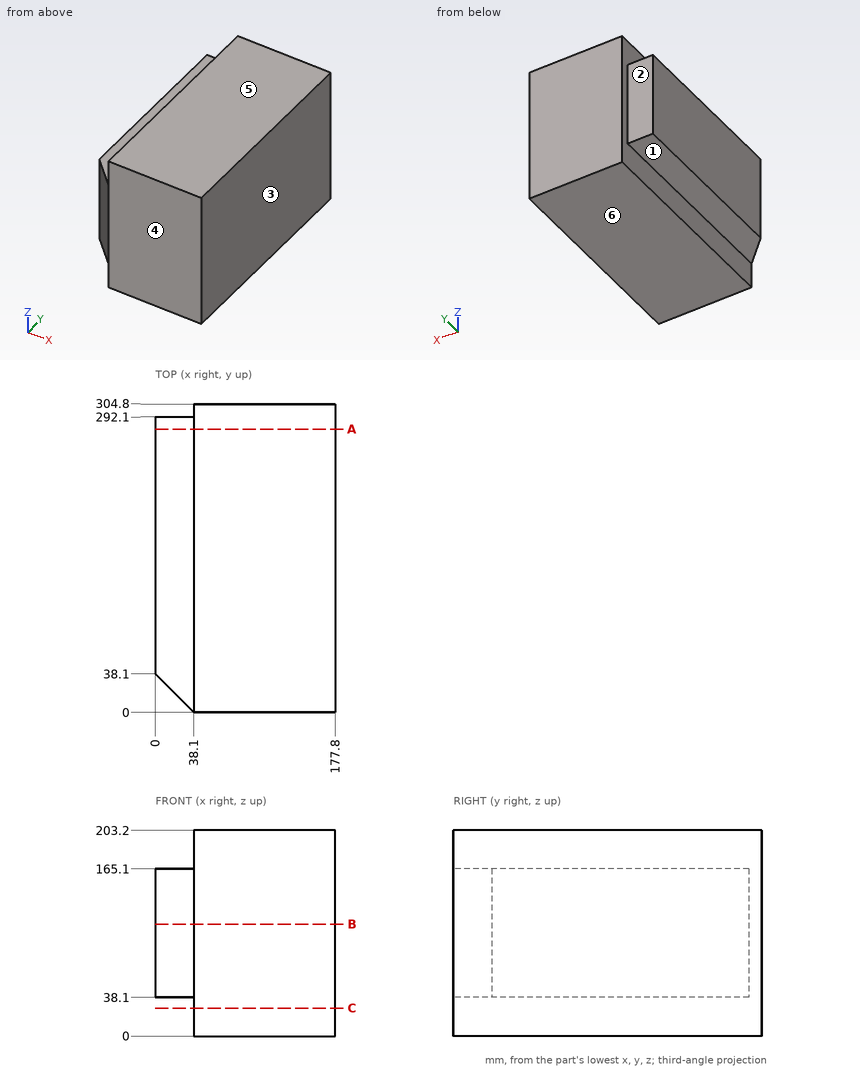
Answer from the drawing. Dimensions are ordinates in mm from the lowest x, y and z of the part. A direction names the side the tool comes from. Round coordinates to 2 decimals unless told otherwise and drop trailing zeros. Loops run counter-clockwise (first coordinate to the right, second up) from the corner with the lowest first, then second, coordinate; pieces in that order, holes last. Notation, with made-up numbers: (-37, 12) - (-32, 12) arc R27 cw to (-32, 33) - close; hole circle Ø6 at (81.5, -9.5). An arc over 180 degrees is marked (long way). Return JSON: item names as keys, results as strings. Group by question number.
1. The mould has two halves that part along Z. Classify the marked faces 4, 5 and 6: pulls with the +Z half, pulls with the -Z half, needs draft (parallel to the pull), parting line crosses it, or undercut.
2. The part is cut by section C-C on z = 27.5. Determine the outline of the cut face in (x, y), then the cut area to 3 significant figures.
3. The part is cut by section B-B on z = 110.5. Determine the outline of the cut face in (x, y), then the cut area to 3 significant figures.
4. Which of the six approach directions +Z, -Z, +X, -X, +Y, -Y give full straight-line access (tool end or side, diameter ignored) to the marked faces 1, 2 and 3?
5. Each of these flat-tipped pins is pushed along its axis until it touches: P1, Ø11.5, axis at x = 24, y = 207, coming from the -Z side; P2, Ø11.5, axis at x = 21.5, z = 93.5, coming from the +Y side. Where does it stop, or does it pass through?
6. Consider probe 1 along X at (y, z) = (199, 177); probe 2 along Z at (x, y) = (11, 184); probe 3 along X at (y, z) = (14.5, 128). Determine where each line is inside the solid, lowest interval first.
7. The part is cut by section A-A on y = 280. Determine the outline of the cut face in (x, z), then the cut area to 3 significant figures.
Resolved:
{
 "1": {"face 4": "needs draft", "face 5": "pulls with the +Z half", "face 6": "pulls with the -Z half"},
 "2": {"outline": "(38.1, 0) - (177.8, 0) - (177.8, 304.8) - (38.1, 304.8) - close", "area": "42,600 mm²"},
 "3": {"outline": "(0, 38.1) - (38.1, 0) - (177.8, 0) - (177.8, 304.8) - (38.1, 304.8) - (38.1, 292.1) - (0, 292.1) - close", "area": "53,000 mm²"},
 "4": {"face 1": "-Z, -X, +Y, -Y", "face 2": "+Z, -Z, -X, +Y", "face 3": "+Z, -Z, +X, +Y, -Y"},
 "5": {"P1": "stops at z = 38.1", "P2": "stops at y = 292.1"},
 "6": {"probe 1": "x = 38.1 to 177.8", "probe 2": "z = 38.1 to 165.1", "probe 3": "x = 23.6 to 177.8"},
 "7": {"outline": "(0, 38.1) - (38.1, 38.1) - (38.1, 0) - (177.8, 0) - (177.8, 203.2) - (38.1, 203.2) - (38.1, 165.1) - (0, 165.1) - close", "area": "33,200 mm²"}
}
